from build123d import *

# Parameters (mm, degrees)
SKETCH_2_R                  = 12.5
EXTRUDE_2_DEPTH             = 250
EXTRUDE_3_DEPTH             = 250
SKETCH_7_R                  = 3.3
CUT_EXTRUDE_1_DEPTH         = 11
HOLE_WIZARD_M51_D           = 5.3
HOLE_WIZARD_M51_DEPTH       = 18
HOLE_WIZARD_M51_CBORE_D     = 10
HOLE_WIZARD_M51_CBORE_DEPTH = 5
HOLE_WIZARD_M51_TIP         = 1.59228064


with BuildPart() as part:
    # Эскиз2 → Бобышка-Вытянуть2 (new body)
    with BuildSketch(Plane.XY):
        Circle(SKETCH_2_R)
    extrude(amount=EXTRUDE_2_DEPTH)

    # Эскиз2<4> → Бобышка-Вытянуть3 (add)
    with BuildSketch(Plane.XY):
        with BuildLine():
            Line((10, -21.97), (4.127670885, -11.798827614))
            ThreePointArc((4.127670885, -11.798827614), (0, -12.5), (-4.127670885, -11.798827614))
            Line((-4.127670885, -11.798827614), (-10, -21.97))
            Line((-10, -21.97), (-32.5, -21.97))
            Line((-32.5, -21.97), (-32.5, -31.97))
            Line((-32.5, -31.97), (-10, -31.97))
            Line((-10, -31.97), (-9.299792462, -30.97))
            Line((-9.299792462, -30.97), (9.299792462, -30.97))
            Line((9.299792462, -30.97), (10, -31.97))
            Line((10, -31.97), (32.5, -31.97))
            Line((32.5, -31.97), (32.5, -21.97))
            Line((32.5, -21.97), (10, -21.97))
        make_face()
    extrude(amount=EXTRUDE_3_DEPTH)

    # Эскиз7 → Вырез-Вытянуть1 (cut, through all)
    with BuildSketch(Plane(origin=(0, -21.97, 0), x_dir=(1, 0, 0), z_dir=(0, 1, 0))):
        with Locations((-18.5, -225)):
            Circle(SKETCH_7_R)
        with Locations((18.5, -225)):
            Circle(SKETCH_7_R)
        with Locations((18.5, -25)):
            Circle(SKETCH_7_R)
        with Locations((-18.5, -25)):
            Circle(SKETCH_7_R)
    extrude(amount=-CUT_EXTRUDE_1_DEPTH, mode=Mode.SUBTRACT)

    # Цековка для винта с внутренним шестигранником M51
    with Locations(Plane(origin=(0, -30.97, 0), x_dir=(-1, 0, 0), z_dir=(0, -1, 0))):
        with Locations((0, -25), (0, -225)):
            CounterBoreHole(HOLE_WIZARD_M51_D / 2, HOLE_WIZARD_M51_CBORE_D / 2, HOLE_WIZARD_M51_CBORE_DEPTH, depth=HOLE_WIZARD_M51_DEPTH)
            with Locations((0, 0, -(HOLE_WIZARD_M51_DEPTH + HOLE_WIZARD_M51_TIP / 2))):  # 118° drill point
                Cone(0, HOLE_WIZARD_M51_D / 2, HOLE_WIZARD_M51_TIP, mode=Mode.SUBTRACT)


solid = part.part
Verification items for the finished model (mm, model axes). A direction names the side the tool comes from. Coordinates: 2 decimals unless noted, no trailing zeros. Order: outer loops, then holes, each group sorted by start corner. A loop starts at its lowest first (then second) coordinate and runs counter-clockwise, first axis right, second up. Notation, with made-up numbers: (-16, 44.25) -> (22, 44.25) arc R11 ccw to (22, 51.25) -> close; hole circle Ø5 at (74.25, -13.75). An arc over 180 degrees is marked (long way). Put each result on its own line as item: value. Start each with the question number.
1. Cross-section at D-D, the plane x = 28. Record the boundary of the cut face in (y, z).
2. Cross-section at C-C, the plane y = 0. Record the boundary of the cut face in (x, z).
3. Cross-section at A-A, the plane x = -18.5. Record the boundary of the cut face in (y, z).
4. Cross-section at B-B, the plane z = 62. Record the boundary of the cut face in (x, y), then the cut area to 3 significant figures.
5. Mould release check, pull along Z, two halves, no side actions. Record for faces 1 (the cylindrical face through (17.78, -26.9, 28.22)), 2 (the flat face through (0, -14, 0)), 3 (the flat face through (-7.02, -16.81, 123.25)): released by +Z, released by -Z, zero draft, split by the parting line, or undercut.
6. Go/stop test with flat-tipped pins: pin 1 Ø6 at (x, z) = (18.5, 225) entering from -Y; pin 2 Ø3 at (y, z) = (7.5, 184) entering from -X; pin 3 Ø4 at (x, y) = (-2, -27) entering from -Z; pin 4 Ø18 at (x, z) = (-23, 148) entering from +Y. Record where each tip stops, or that it passes through.
7. Material ranges on L1, parallel to X at y = -25.75, z = 225; L2, parallel to Z at x = 18, y = -28; L3, parallel to Z at x = 0, y = -22, recorded low to high. Write a range as [from, to].
8. Access from +Z, -Z, +X, -X, +Y, -Y to the whole of each face (thin tool, end or side, straight path). Record for faces 4 (the flat face through (-2, -25.97, 27)), 5 (the flat face through (21, -31.97, 123)), 6 (the flat face through (0, -30.97, 123)).
Computed:
1. outline: (-31.97, 0) -> (-21.97, 0) -> (-21.97, 250) -> (-31.97, 250) -> close
2. outline: (-12.5, 0) -> (12.5, 0) -> (12.5, 250) -> (-12.5, 250) -> close
3. outline: (-31.97, 0) -> (-21.97, 0) -> (-21.97, 21.7) -> (-31.97, 21.7) -> close; (-31.97, 28.3) -> (-21.97, 28.3) -> (-21.97, 221.7) -> (-31.97, 221.7) -> close; (-31.97, 228.3) -> (-21.97, 228.3) -> (-21.97, 250) -> (-31.97, 250) -> close
4. outline: (-32.5, -31.97) -> (-10, -31.97) -> (-9.3, -30.97) -> (9.3, -30.97) -> (10, -31.97) -> (32.5, -31.97) -> (32.5, -21.97) -> (10, -21.97) -> (4.13, -11.8) arc R12.5 ccw (long way) to (-4.13, -11.8) -> (-10, -21.97) -> (-32.5, -21.97) -> close
4. area: 1,260 mm2
5. face 1: undercut
5. face 2: released by -Z
5. face 3: zero draft
6. pin 1: through
6. pin 2: x = -10.97
6. pin 3: z = 0
6. pin 4: y = -21.97
7. L1: [-32.5, -21.8], [-15.2, -2.65], [2.65, 15.2], [21.8, 32.5]
7. L2: [0, 21.74], [28.26, 221.74], [228.26, 250]
7. L3: [0, 22.35], [27.65, 222.35], [227.65, 250]
8. face 4: -Y
8. face 5: +Z, -Z, +X, -X, -Y
8. face 6: +Z, -Z, -Y
